from build123d import *

# Parameters (mm, degrees)
IZIM1_R                     = 55
Y_KSEKLIK_EKSTR_ZYON1_DEPTH = 42
IZIM4_R                     = 45
Y_KSEKLIK_EKSTR_ZYON2_DEPTH = 30
IZIM5_R                     = 30
IZIM5_R_2                   = 27
KES_EKSTR_ZYON1_DEPTH       = 2
IZIM6_R                     = 35
Y_KSEKLIK_EKSTR_ZYON3_DEPTH = 72
IZIM7_R                     = 22.5
IZIM7_R_2                   = 17.5
KES_EKSTR_ZYON2_DEPTH       = 2
IZIM18_R                    = 3
KES_EKSTR_ZYON3_DEPTH       = 4
KUBBE1_FACE_RADIUS          = 17.5
KUBBE1_HEIGHT               = 10
KUBBE2_FACE_RADIUS          = 27
KUBBE2_HEIGHT               = 10
IZIM19_R                    = 15
Y_KSEKLIK_EKSTR_ZYON4_DEPTH = 20


with BuildPart() as part:
    # Çizim1 → Yükseklik-Ekstrüzyon1 (new body)
    with BuildSketch(Plane(origin=(0, 0, 0), x_dir=(1, 0, 0), z_dir=(0, 1, 0))):
        with Locations(Location((0, 0, 0), (0, 0, 90))):
            Circle(IZIM1_R)
    extrude(amount=Y_KSEKLIK_EKSTR_ZYON1_DEPTH)

    # Çizim4 → Yükseklik-Ekstrüzyon2 (add)
    with BuildSketch(Plane(origin=(0, 42, 0), x_dir=(1, 0, 0), z_dir=(0, 1, 0))):
        with Locations(Location((0, 0, 0), (0, 0, 270))):
            Circle(IZIM4_R)
    extrude(amount=Y_KSEKLIK_EKSTR_ZYON2_DEPTH)

    # Çizim5 → Kes-Ekstrüzyon1 (cut)
    with BuildSketch(Plane(origin=(0, 72, 0), x_dir=(1, 0, 0), z_dir=(0, 1, 0))):
        with Locations(Location((0, 0, 0), (0, 0, 270))):
            Circle(IZIM5_R)
        with Locations(Location((0, 0, 0), (0, 0, 270))):
            Circle(IZIM5_R_2, mode=Mode.SUBTRACT)
    extrude(amount=-KES_EKSTR_ZYON1_DEPTH, mode=Mode.SUBTRACT)



with BuildPart() as body_2:
    # Çizim6 → Yükseklik-Ekstrüzyon3 (new body)
    with BuildSketch(Plane(origin=(0, 72, 0), x_dir=(1, 0, 0), z_dir=(0, 1, 0))):
        with Locations(Location((-300, 0, 0), (0, 0, 270))):
            Circle(IZIM6_R)
    extrude(amount=-Y_KSEKLIK_EKSTR_ZYON3_DEPTH)

    # Çizim7 → Kes-Ekstrüzyon2 (cut)
    with BuildSketch(Plane(origin=(0, 72, 0), x_dir=(1, 0, 0), z_dir=(0, 1, 0))):
        with Locations(Location((-300, 0, 0), (0, 0, 270))):
            Circle(IZIM7_R)
        with Locations(Location((-300, 0, 0), (0, 0, 270))):
            Circle(IZIM7_R_2, mode=Mode.SUBTRACT)
    extrude(amount=-KES_EKSTR_ZYON2_DEPTH, mode=Mode.SUBTRACT)


with BuildPart() as part_1:
    add(part.part)

    add(body_2.part)  # Loft1 merges body 2
    # Çizim17 for Loft1 → Loft1 section 0
    with BuildSketch(Plane(origin=(0, 0, 0), x_dir=(0, 0, -1), z_dir=(1, 0, 0))):
        with BuildLine():
            Line((-39.5, 0), (39.5, 0))
            # circular arc as an exact rational Bezier (weights 1, cos(half-angle), 1)
            Bezier((39.5, 0), (0, 247.471747323), (-39.5, 0), weights=[1, 0.157619003, 1])
        make_face()
    # Çizim16 for Loft1 → Loft1 section 1
    with BuildSketch(Plane(origin=(-300, 0, 0), x_dir=(0, 0, -1), z_dir=(1, 0, 0))):
        with BuildLine():
            Line((-25, 0), (25, 0))
            Bezier((25, 0), (0, 87.517505252), (-25, 0), weights=[1, 0.274670324, 1])
        make_face()
    loft()

    # Çizim18 → Kes-Ekstrüzyon3 (cut)
    with BuildSketch(Plane(origin=(0, 42, 0), x_dir=(1, 0, 0), z_dir=(0, 1, 0))):
        with Locations(Location((-25.147379783, 44.942844703, 0), (0, 0, 270))):
            Circle(IZIM18_R)
        with Locations(Location((-3.157036788, 51.403143082, 0), (0, 0, 270))):
            Circle(IZIM18_R)
        with Locations(Location((19.458596062, 47.682418555, 0), (0, 0, 270))):
            Circle(IZIM18_R)
        with Locations(Location((38.220215318, 34.517606247, 0), (0, 0, 270))):
            Circle(IZIM18_R)
        with Locations(Location((49.41185219, 14.516158691, 0), (0, 0, 270))):
            Circle(IZIM18_R)
        with Locations(Location((50.816865739, -8.360392123, 0), (0, 0, 270))):
            Circle(IZIM18_R)
        with Locations(Location((42.156975801, -29.581064743, 0), (0, 0, 270))):
            Circle(IZIM18_R)
        with Locations(Location((25.147379783, -44.942844703, 0), (0, 0, 270))):
            Circle(IZIM18_R)
        with Locations(Location((3.157036788, -51.403143082, 0), (0, 0, 270))):
            Circle(IZIM18_R)
        with Locations(Location((-19.458596062, -47.682418555, 0), (0, 0, 270))):
            Circle(IZIM18_R)
        with Locations(Location((-38.220215318, -34.517606247, 0), (0, 0, 270))):
            Circle(IZIM18_R)
        with Locations(Location((-49.41185219, -14.516158691, 0), (0, 0, 270))):
            Circle(IZIM18_R)
        with Locations(Location((-50.816865739, 8.360392123, 0), (0, 0, 270))):
            Circle(IZIM18_R)
        with Locations(Location((-42.156975801, 29.581064743, 0), (0, 0, 270))):
            Circle(IZIM18_R)
    extrude(amount=-KES_EKSTR_ZYON3_DEPTH, mode=Mode.SUBTRACT)

    # Kubbe1: a dome of height H over a round flat face of radius A is a cap of a sphere of radius (A * A + H * H) / (2 * H)
    kubbe1_r = (KUBBE1_FACE_RADIUS * KUBBE1_FACE_RADIUS + KUBBE1_HEIGHT * KUBBE1_HEIGHT) / (2 * KUBBE1_HEIGHT)
    kubbe1_base = Plane((-300, 72, 0), z_dir=(0, 1, 0))
    with Locations(kubbe1_base.offset(KUBBE1_HEIGHT - kubbe1_r)):
        kubbe1_ball = Sphere(kubbe1_r, mode=Mode.PRIVATE)
    add(split(kubbe1_ball, bisect_by=kubbe1_base, keep=Keep.TOP, mode=Mode.PRIVATE))

    # Kubbe2: a dome of height H over a round flat face of radius A is a cap of a sphere of radius (A * A + H * H) / (2 * H)
    kubbe2_r = (KUBBE2_FACE_RADIUS * KUBBE2_FACE_RADIUS + KUBBE2_HEIGHT * KUBBE2_HEIGHT) / (2 * KUBBE2_HEIGHT)
    kubbe2_base = Plane((0, 72, 0), z_dir=(0, 1, 0))
    with Locations(kubbe2_base.offset(KUBBE2_HEIGHT - kubbe2_r)):
        kubbe2_ball = Sphere(kubbe2_r, mode=Mode.PRIVATE)
    add(split(kubbe2_ball, bisect_by=kubbe2_base, keep=Keep.TOP, mode=Mode.PRIVATE))

    # Çizim19 → Yükseklik-Ekstrüzyon4 (add)
    with BuildSketch(Plane.XZ):
        with Locations(Location((-300, 0, 0), (0, 0, 90))):
            Circle(IZIM19_R)
        with Locations(Location((0, 0, 0), (0, 0, 90))):
            Circle(IZIM19_R)
    extrude(amount=Y_KSEKLIK_EKSTR_ZYON4_DEPTH)


solid = part_1.part
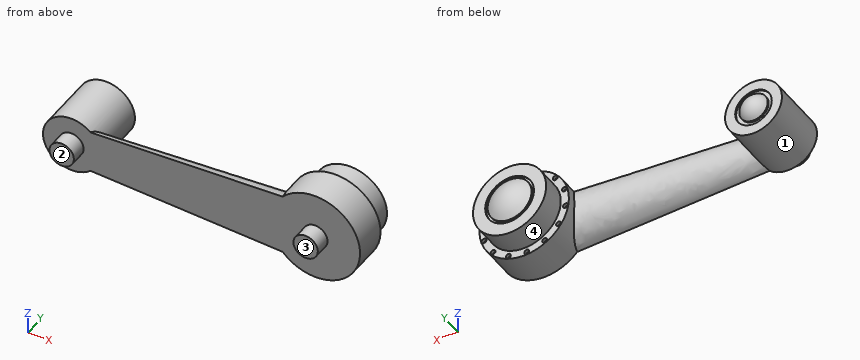
Could you check a few things on this model? Use its own coordinates, in mm. Face numbers are marked on the shaded views. A direction names the side the tool comes from. Give positions to 0.01 mm unless a question says otherwise; leave off trailing zeros. Order: outer loops, then holes, each group sorted by start corner. A loop starts at its lowest first (then second) coordinate and runs counter-clockwise, first axis right, second up. Notation, with made-up numbers: M 11,42 L 30,42 A15 cw 30,60 Z; hole C 3,80 d4. An arc over 180 degrees is marked long. One line per question, with ' | ' between items.
1. If I drill on line 1 (Y direction, x = -175, z = -29); line 2 (X direction, y = 57.5, z = 14); line 3 (X direction, y = 54, z = -3), over which ranges is the centre line in solid material (lowest first)?
Results:
line 1: 0 to 6.21 | line 2: -332.08 to -267.92, -42.77 to 42.77 | line 3: -334.87 to -265.13, -44.9 to 44.9
2. I want a section at A-A (y = -7). List the corners of the cut face in (x, z) for me.
Results:
outline: C -300,0 d30; C 0,0 d30
3. I want a section at B-B (x = -300). List the corners of the cut face in (y, z) for me (1 decimal), and give its area (3 significant figures).
Results:
outline: M -20,-15 L 0,-15 L 0,-35 L 72,-35 L 72,-22.5 L 70,-22.5 L 70,-17.5 L 72,-17.5 A20.3 ccw 72,17.5 L 70,17.5 L 70,22.5 L 72,22.5 L 72,35 L 0,35 L 0,15 L -20,15 Z | area: 5,870 mm²
4. We'd pull the mould along X, two halves only. Please class the marked faces 1 and 2: +X half, -X half, draft (parallel to the pull), parting line (faces both ways), or undercut.
Results:
face 1: undercut | face 2: draft
5. I'm going to push flat-ended pins straight in: pin 1 (1.5 mm diameter, centred on y = -6.5, z = 14.5, fed in from +X); pin 2 (3 mm diameter, centred on y = 19.5, z = -33, fed in from +X); pin 3 (5 mm diameter, centred on x = -50.82, z = -8.36, fed in from -Y). Where does each tip first touch, or does it pass through?
Results:
pin 1: x = 5.99 | pin 2: x = 45.09 | pin 3: y = 0
6. For the marked faces 3 and 4, which set-ups out of +Z, -Z, +X, -X, +Y, -Y let a thin tool reach every point of the face, with its end or its side?
Results:
face 3: +Z, -Z, +X, -X, -Y | face 4: +Y
